from build123d import *

# Parameters (mm, degrees)
BOSS_EXTRUDE1_DEPTH = 6


with BuildPart() as part:
    # Model → Boss-Extrude1 (new body)
    with BuildSketch(Plane.XY):
        with BuildLine():
            Line((3624.683047417, 1289.903027574), (3615.254475988, 1289.903027574))
            Line((3615.254475988, 1289.903027574), (3615.254475988, 1292.903027574))
            Line((3615.254475988, 1292.903027574), (3609.254475988, 1292.903027574))
            Line((3609.254475988, 1292.903027574), (3609.254475988, 1289.903027574))
            Line((3609.254475988, 1289.903027574), (3603.254475988, 1289.903027574))
            Line((3603.254475988, 1289.903027574), (3603.254475988, 1292.903027574))
            Line((3603.254475988, 1292.903027574), (3597.254475988, 1292.903027574))
            Line((3597.254475988, 1292.903027574), (3597.254475988, 1289.903027574))
            Line((3597.254475988, 1289.903027574), (3587.82590456, 1289.903027574))
            ThreePointArc((3587.82590456, 1289.903027574), (3606.254475988, 1308.331599003), (3624.683047417, 1289.903027574))
        make_face()
    extrude(amount=BOSS_EXTRUDE1_DEPTH)


solid = part.part
Here's how the part is built. I have some questions about the finished solid (model axes, mm). A direction names the side the tool comes from. Give positions to 0.01 mm unless a question says otherwise; leave off trailing zeros. Order: outer loops, then holes, each group sorted by start corner. A loop starts at its lowest first (then second) coordinate and runs counter-clockwise, first axis right, second up. Notation, with made-up numbers: M -33.5,53 L 0.5,53 A19 ccw 0.5,87 Z; hole C 21.5,-10 d11. An arc over 180 degrees is marked long. Answer as a JSON object with one key per item and string values. Group by question number.
1) I'm going to push flat-ended pins straight in: pin 1 Ø3 at (y, z) = (1298, 4) entering from +X; pin 2 Ø1.5 at (y, z) = (1291, 2) entering from +X; pin 3 Ø1.5 at (y, z) = (1291.5, 3) entering from -X. Where does each tip first touch, or does it pass through?
2) Please list where these lines run through material, in increasing order: L1, parallel to X at y = 1292.75, z = 4.55; L2, parallel to X at y = 1303.5, z = 2.1; L3, parallel to X at y = 1301, z = 5.5. Write a range as [from, to].
3) On a 3-axis mill with a long thin cutter (end or side, diameter ignored), from which of +Z, -Z, +X, -X, +Y, -Y can I reach the whole of each face in a straight line? I mean faces 1 (the flat face through (3603.254, 1291, 3)), 2 (the flat face through (3620, 1289.903, 3)). Say none if no direction works.
4) Suppose I cut it at B-B, the plane x = 3619. Write out the boundary of the cut face in (y, z), plus the area to 3 significant figures.
5) Suppose I cut it at C-C, the plane y = 1305.75. Write out the boundary of the cut face in (x, z), plus the area to 3 significant figures.
Results found:
{
 "1": {"pin 1": "x = 3623.46", "pin 2": "x = 3624.68", "pin 3": "x = 3587.85"},
 "2": {"L1": "[3588.05, 3597.25], [3603.25, 3609.25], [3615.25, 3624.46]", "L2": "[3593.82, 3618.69]", "L3": "[3591.54, 3620.97]"},
 "3": {"face 1": "+Z, -Z, -Y", "face 2": "+Z, -Z, +X, -X, -Y"},
 "4": {"outline": "M 1289.9,0 L 1303.21,0 L 1303.21,6 L 1289.9,6 Z", "area": "79.9 mm²"},
 "5": {"outline": "M 3596.85,0 L 3615.66,0 L 3615.66,6 L 3596.85,6 Z", "area": "113 mm²"}
}
